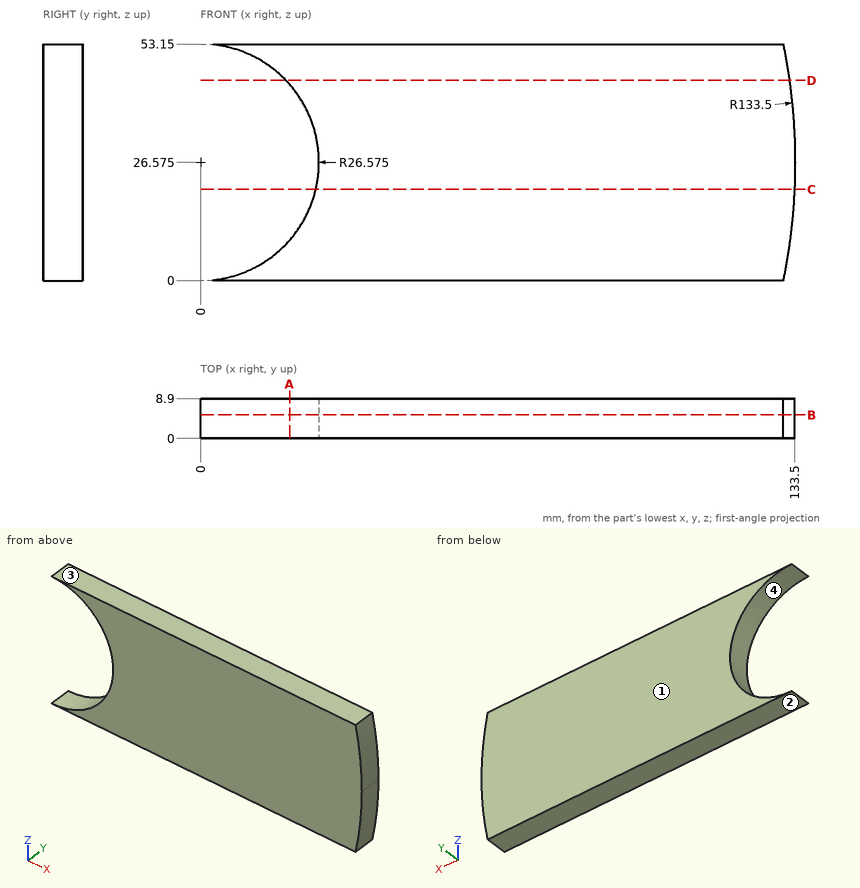
Source: three-view drawing plus pictorial views. Frame: mm from the lowest corner of the part. Coordinates: 2 decimals unless noted, no trailing zeros. Loops run counter-clockwise (first coordinate to the right, second up) from the corner with the lowest first, then second, coordinate; pieces in that order, holes last. Notation, with made-up numbers: (71, 70.25) -> (120, 70.25) arc R29 ccw to (120, 103.25) -> close; hole circle Ø3 at (7.5, -1). An arc over 180 degrees is marked (long way). One line per item, written item: value.
(1) Cut plane B-B (y = 5.25). Output: boundary loops of the cut face in (x, z) (3 decimals), then the cut area to 3 significant figures.
Answer below:
outline: (0, 0) -> (130.828, 0) arc R133.5 ccw to (130.828, 53.15) -> (0, 53.15) arc R26.575 cw to start
area: 5,940 mm2
(2) Ray query, line 1 along X through (y, z) = (6.5, 15.5); line 2 along X through (y, z) = (2.5, 47.5). Return the intervals inside material, ascending.
Answer below:
line 1: x = 24.16 to 133.04
line 2: x = 16.38 to 131.85
(3) Cut plane D-D (z = 45). Output: boundary loops of the cut face in (x, y), then the cut area to 3 significant figures.
Answer below:
outline: (19.15, 0) -> (132.22, 0) -> (132.22, 8.9) -> (19.15, 8.9) -> close
area: 1,010 mm2
(4) Draft query along Z for the marked faces 1, 2, 3 and 4. Return one class per face: pulls with the +Z half, pulls with the -Z half, needs draft (parallel to the pull), parting line crosses it, or undercut.
Answer below:
face 1: needs draft
face 2: pulls with the -Z half
face 3: pulls with the +Z half
face 4: undercut
(5) Pin query (flat end, axial travel): pin 1 Ø4 at (x, z) = (90, 18.5) entering from -Y; pin 2 Ø1.5 at (y, z) = (4.5, 33) entering from -X; pin 3 Ø3 at (y, z) = (7, 25) entering from -X. Return the tip coordinate at first contact, or that it passes through.
Answer below:
pin 1: stops at y = 0
pin 2: stops at x = 25.59
pin 3: stops at x = 26.4
(6) Cut plane C-C (z = 20.5). Output: boundary loops of the cut face in (x, y), then the cut area to 3 significant figures.
Answer below:
outline: (25.87, 0) -> (133.36, 0) -> (133.36, 8.9) -> (25.87, 8.9) -> close
area: 957 mm2
(7) Cut plane A-A (x = 20). Output: boundary loops of the cut face in (y, z), then the cut area to 3 significant figures.
Answer below:
outline: (0, 0) -> (8.9, 0) -> (8.9, 9.08) -> (0, 9.08) -> close; (0, 44.07) -> (8.9, 44.07) -> (8.9, 53.15) -> (0, 53.15) -> close
area: 162 mm2
